```python
from build123d import *

# Parameters (mm, degrees)
F0_R     = 2.6035
F1_DEPTH = 317.5


# Not quite as in the source:
# - ends of sketch curves that miss each other by under 0.0002 mm in the source are joined


with BuildPart() as f1:
    # F0 (on Front) → F1 (new body, symmetric)
    with BuildSketch(Plane.XZ):
        with BuildLine():
            ThreePointArc((-120.045226, 66.1162), (-119.5372260057, 65.6082762), (-120.0450736, 65.1002000229))
            ThreePointArc((-120.0450736, 65.1002000229), (-119.4277485161, 63.5840774839), (-117.9116260074, 62.9667530175))
            ThreePointArc((-117.9116260074, 62.9667530175), (-117.4035498, 63.4745999943), (-116.895626, 62.9666))
            Line((-116.895626, 62.9666), (-113.6783096, 62.9666))
            ThreePointArc((-113.6783096, 62.9666), (-113.1703096, 63.4746), (-112.6623096, 62.9666))
            Line((-112.6623096, 62.9666), (-111.688626, 62.9666))
            ThreePointArc((-111.688626, 62.9666), (-110.583726, 64.0715), (-111.688626, 65.1764))
            Line((-111.688626, 65.1764), (-113.8200162, 65.1764))
            ThreePointArc((-113.8200162, 65.1764), (-114.758677805, 65.8035936327), (-114.5384366897, 66.9108204897))
            Line((-114.5384366897, 66.9108204897), (-111.2083882, 70.2408552))
            ThreePointArc((-111.2083882, 70.2408552), (-110.1783528978, 70.9291175157), (-108.963333, 71.1708))
            Line((-108.963333, 71.1708), (-105.727119, 71.1708))
            ThreePointArc((-105.727119, 71.1708), (-104.5120991022, 70.9291175157), (-103.4820549697, 70.2408640303))
            Line((-103.4820549697, 70.2408640303), (-100.1520222, 66.9108136))
            ThreePointArc((-100.1520222, 66.9108136), (-99.931774195, 65.8035936327), (-100.8704358, 65.1764))
            Line((-100.8704358, 65.1764), (-103.001826, 65.1764))
            ThreePointArc((-103.001826, 65.1764), (-104.106726, 64.0715), (-103.001826, 62.9666))
            Line((-103.001826, 62.9666), (-102.0281424, 62.9666))
            ThreePointArc((-102.0281424, 62.9666), (-101.5201424, 63.4746), (-101.0121424, 62.9666))
            Line((-101.0121424, 62.9666), (-97.794826, 62.9666))
            ThreePointArc((-97.794826, 62.9666), (-97.2869022, 63.4745999943), (-96.7788260229, 62.9667524))
            ThreePointArc((-96.7788260229, 62.9667524), (-95.2627034839, 63.5840774839), (-94.6453790175, 65.1001999926))
            ThreePointArc((-94.6453790175, 65.1001999926), (-95.1532259943, 65.6082762), (-94.645226, 66.1162))
            Line((-94.645226, 66.1162), (-94.645226, 69.3335164))
            ThreePointArc((-94.645226, 69.3335164), (-95.153226, 69.8415164), (-94.645226, 70.3495164))
            Line((-94.645226, 70.3495164), (-94.645226, 71.3232))
            ThreePointArc((-94.645226, 71.3232), (-95.750126, 72.4281), (-96.855026, 71.3232))
            Line((-96.855026, 71.3232), (-96.855026, 69.1918098))
            ThreePointArc((-96.855026, 69.1918098), (-97.4822196327, 68.253148195), (-98.5894464897, 68.4733893103))
            Line((-98.5894464897, 68.4733893103), (-101.9194812, 71.8034378))
            ThreePointArc((-101.9194812, 71.8034378), (-102.6077435157, 72.8334731022), (-102.849426, 74.048493))
            Line((-102.849426, 74.048493), (-102.849426, 77.284707))
            ThreePointArc((-102.849426, 77.284707), (-102.6077435157, 78.4997268978), (-101.9194900303, 79.5297710303))
            Line((-101.9194900303, 79.5297710303), (-98.5894396, 82.8598038))
            ThreePointArc((-98.5894396, 82.8598038), (-97.4822196327, 83.080051805), (-96.855026, 82.1413902))
            Line((-96.855026, 82.1413902), (-96.855026, 80.01))
            ThreePointArc((-96.855026, 80.01), (-95.750126, 78.9051), (-94.645226, 80.01))
            Line((-94.645226, 80.01), (-94.645226, 80.9836836))
            ThreePointArc((-94.645226, 80.9836836), (-95.153226, 81.4916836), (-94.645226, 81.9996836))
            Line((-94.645226, 81.9996836), (-94.645226, 85.217))
            ThreePointArc((-94.645226, 85.217), (-95.1532259943, 85.7249238), (-94.6453784, 86.2329999771))
            ThreePointArc((-94.6453784, 86.2329999771), (-95.2627034839, 87.7491225161), (-96.7788259926, 88.3664469825))
            ThreePointArc((-96.7788259926, 88.3664469825), (-97.2869022, 87.8586000057), (-97.794826, 88.3666))
            Line((-97.794826, 88.3666), (-101.0121424, 88.3666))
            ThreePointArc((-101.0121424, 88.3666), (-101.5201424, 87.8586), (-102.0281424, 88.3666))
            Line((-102.0281424, 88.3666), (-103.001826, 88.3666))
            ThreePointArc((-103.001826, 88.3666), (-104.106726, 87.2617), (-103.001826, 86.1568))
            Line((-103.001826, 86.1568), (-100.8704358, 86.1568))
            ThreePointArc((-100.8704358, 86.1568), (-99.931774195, 85.5296063673), (-100.1520153103, 84.4223795103))
            Line((-100.1520153103, 84.4223795103), (-103.4820638, 81.0923448))
            ThreePointArc((-103.4820638, 81.0923448), (-104.5120991022, 80.4040824843), (-105.727119, 80.1624))
            Line((-105.727119, 80.1624), (-108.963333, 80.1624))
            ThreePointArc((-108.963333, 80.1624), (-110.1783528978, 80.4040824843), (-111.2083970303, 81.0923359697))
            Line((-111.2083970303, 81.0923359697), (-114.5384298, 84.4223864))
            ThreePointArc((-114.5384298, 84.4223864), (-114.758677805, 85.5296063673), (-113.8200162, 86.1568))
            Line((-113.8200162, 86.1568), (-111.688626, 86.1568))
            ThreePointArc((-111.688626, 86.1568), (-110.583726, 87.2617), (-111.688626, 88.3666))
            Line((-111.688626, 88.3666), (-112.6623096, 88.3666))
            ThreePointArc((-112.6623096, 88.3666), (-113.1703096, 87.8586), (-113.6783096, 88.3666))
            Line((-113.6783096, 88.3666), (-116.895626, 88.3666))
            ThreePointArc((-116.895626, 88.3666), (-117.4035498, 87.8586000057), (-117.9116259771, 88.3664476))
            ThreePointArc((-117.9116259771, 88.3664476), (-119.4277485161, 87.7491225161), (-120.0450729825, 86.2330000074))
            ThreePointArc((-120.0450729825, 86.2330000074), (-119.5372260057, 85.7249238), (-120.045226, 85.217))
            Line((-120.045226, 85.217), (-120.045226, 81.9996836))
            ThreePointArc((-120.045226, 81.9996836), (-119.537226, 81.4916836), (-120.045226, 80.9836836))
            Line((-120.045226, 80.9836836), (-120.045226, 80.01))
            ThreePointArc((-120.045226, 80.01), (-118.940326, 78.9051), (-117.835426, 80.01))
            Line((-117.835426, 80.01), (-117.835426, 82.1413902))
            ThreePointArc((-117.835426, 82.1413902), (-117.2082323673, 83.080051805), (-116.1010055103, 82.8598106897))
            Line((-116.1010055103, 82.8598106897), (-112.7709708, 79.5297622))
            ThreePointArc((-112.7709708, 79.5297622), (-112.0827084843, 78.4997268978), (-111.841026, 77.284707))
            Line((-111.841026, 77.284707), (-111.841026, 74.048493))
            ThreePointArc((-111.841026, 74.048493), (-112.0827084843, 72.8334731022), (-112.7709619697, 71.8034289697))
            Line((-112.7709619697, 71.8034289697), (-116.1010124, 68.4733962))
            ThreePointArc((-116.1010124, 68.4733962), (-117.2082323673, 68.253148195), (-117.835426, 69.1918098))
            Line((-117.835426, 69.1918098), (-117.835426, 71.3232))
            ThreePointArc((-117.835426, 71.3232), (-118.940326, 72.4281), (-120.045226, 71.3232))
            Line((-120.045226, 71.3232), (-120.045226, 70.3495164))
            ThreePointArc((-120.045226, 70.3495164), (-119.537226, 69.8415164), (-120.045226, 69.3335164))
            Line((-120.045226, 69.3335164), (-120.045226, 66.1162))
        make_face()
        with Locations((-107.345226, 75.6666)):
            Circle(F0_R, mode=Mode.SUBTRACT)
    extrude(amount=F1_DEPTH, both=True)


solid = f1.part
```
The listing builds one solid part. Answer for the finished solid, in the listing's coordinates (mm). Give positions to 0.01 mm unless a question says otherwise; leave off trailing zeros. Answer as CSV lines item,"result". Start each with the question number.
Item 1: Find the intervals of material crossed by line 1 (X direction, y = 242, z = 69.75); line 2 (X direction, y = 27, z = 79.5); line 3 (Z direction, x = -111.25, y = 153), in increasing order. Write a range as from..to.
Item 2: The mould has two halves that part along Y. Classify faces 1 (the face through (-108, -317.5, 79)), 2 (the face through (-108, 317.5, 79)): +Y half, -Y half, draft (parallel to the pull), parting line (faces both ways), or undercut.
Item 3: Each of these flat-tipped pins is pushed along its axis until it touches: pin 1 (3.5 mm diameter, centred on y = -8, z = 76.5, fed in from +X); pin 2 (2.5 mm diameter, centred on x = -108, y = -27, fed in from +Z); pin 3 (2.5 mm diameter, centred on y = 145.5, z = 75, fed in from -X). Where does it stop, or does it pass through?
Found:
1,line 1,"x = -119.55..-117.84, -114.82..-111.7, -102.99..-99.87, -96.86..-95.14"
1,line 2,"x = -119.92..-117.96, -112.74..-101.95, -96.73..-94.77"
1,line 3,"z = 63.06..65.09, 70.2..81.13, 86.25..88.28"
2,face 1,"-Y half"
2,face 2,"+Y half"
3,pin 1,"stops at x = -102.7"
3,pin 2,"stops at z = 80.18"
3,pin 3,"stops at x = -111.86"
